The drawing under review shows one solid part. Ordinate dimensions are in mm from its lowest x, y, z. A direction names the side the tool comes from. Coordinates: 2 decimals unless noted, no trailing zeros. Write each loop counter-clockwise with the first axis right and the second up, starting at its lowest first coordinate (ties: lowest second). Pieces come first, ordered by that corner, then holes. Notation, with made-up numbers: (-36, -39.5) - (-22, -39.5) arc R28 cw to (-22, -4.5) - close; hole circle Ø8 at (-33, -15.75). An arc over 180 degrees is marked (long way). Answer as CSV lines item,"result". Start each with the question number.
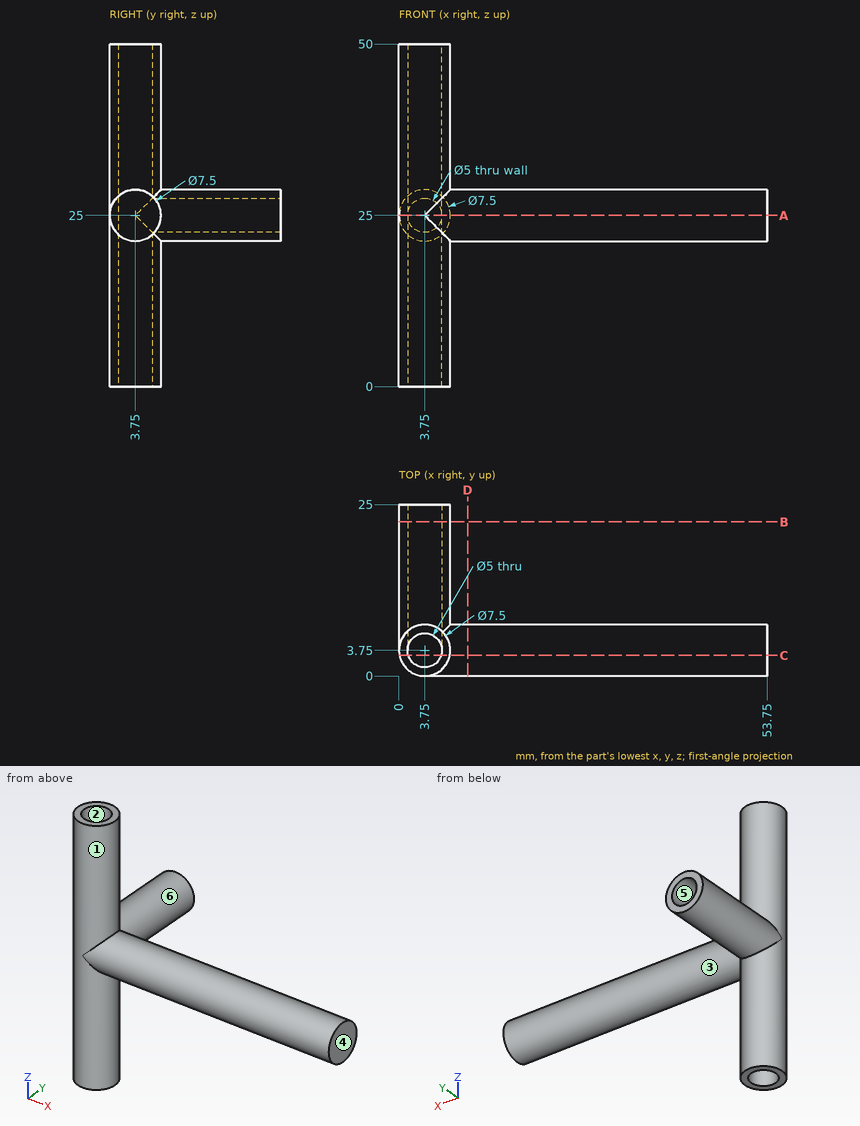
(1) Add section A-A on z = 25. Give the boundary of the cut face in (x, y).
(2) Add section D-D on x = 10. Give the boundary of the cut face in (y, z), then the cut area to 3 significant figures.
(3) Wall thickness on line 1 (X direction, y = 3.75, z = 12); line 2 (X direction, y = 3.75, z = 24.5); line 3 (Z direction, x = 3.75, y = 20.75): over which ranges is each line inside the solid? List them lowest first.
(4) The part is to be moulded in two halves that separate along Z. For the marked faces 4, 5 and 6, say which applies: released by +Z, released by -Z, zero draft, split by the parting line, or undercut.
(5) For the marked faces 1, 2 and 3, list the 3-axis set-ups (+Z, -Z, +X, -X, +Y, -Y) from which the entire face can be reached by the end or side of a thin tool; tool diameter is ignored.
(6) For pin 1 (3 mm diameter, centred on x = 8.5, y = 17.5, fed in from +Z); pin 2 (12 mm diameter, centred on x = 11.5, z = 16.5, fed in from -Y); pin 3 (8 mm diameter, centred on x = 31.5, z = 21, fed in from +Y); pin 4 (1 mm diameter, centred on y = 9.5, z = 32.5, fed in from -X), all flat-tipped, find the tip position at first contact; note any pin that passes through.
(7) Add section B-B on y = 22.5. Give the boundary of the cut face in (x, z).
(8) Add section C-C on y = 3. Give the boundary of the cut face in (x, z).
Reported:
1,outline,"(0, 3.75) arc R3.75 ccw to (3.75, 0) - (53.75, 0) - (53.75, 7.5) - (7.5, 7.5) - (7.5, 25) - (6.25, 25) - (6.25, 3.75) arc R2.5 cw to (1.25, 3.75) - (1.25, 25) - (0, 25) - close"
2,outline,"circle Ø7.5 at (3.75, 25)"
2,area,"44.2 mm²"
3,line 1,"0 to 1.25, 6.25 to 7.5"
3,line 2,"0 to 1.25, 6.25 to 53.75"
3,line 3,"21.25 to 22.5, 27.5 to 28.75"
4,face 4,"zero draft"
4,face 5,"undercut"
4,face 6,"split by the parting line"
5,face 1,"none"
5,face 2,"+Z, -Z"
5,face 3,"+X"
6,pin 1,"z = 26.87"
6,pin 2,"y = 0.43"
6,pin 3,"y = 7.5"
6,pin 4,"through"
7,outline,"circle Ø7.5 at (3.75, 25); hole circle Ø5 at (3.75, 25)"
8,outline,"(0.08, 0) - (1.37, 0) - (1.37, 50) - (0.08, 50) - close; (6.13, 0) - (7.42, 0) - (7.42, 21.33) - (53.75, 21.33) - (53.75, 28.67) - (7.42, 28.67) - (7.42, 50) - (6.13, 50) - close"
